```python
from build123d import *

# Parameters (mm, degrees)
SKETCH1_R               = 30.5
BOSS_EXTRUDE1_DEPTH     = 3
CUT_EXTRUDE1_DEPTH      = 95.663789341
CUT_EXTRUDE1_DEPTH_BACK = 95.663789341
SKETCH10_R              = 4
CUT_EXTRUDE2_DEPTH      = 104.861605143
SKETCH11_R              = 21
CUT_EXTRUDE3_DEPTH      = 93.207554018
FILLET1_R               = 5
FILLET2_R               = 5
FILLET3_R               = 5


with BuildPart() as part:
    # Sketch1 → Boss-Extrude1 (new body)
    with BuildSketch(Plane(origin=(0, 0, 0), x_dir=(1, 0, 0), z_dir=(0, 1, 0))):
        Circle(SKETCH1_R)
        with BuildLine():
            Line((22, 21.124630174), (22, 28.495613698))
            ThreePointArc((22, 28.495613698), (0, 36), (-22, 28.495613698))
            Line((-22, 28.495613698), (-22, 21.124630174))
            ThreePointArc((-22, 21.124630174), (0, 30.5), (22, 21.124630174))
        make_face()
    extrude(amount=BOSS_EXTRUDE1_DEPTH)

    # Sketch2 → Loft1 section 0
    with BuildSketch(Plane(origin=(0, 3, 0), x_dir=(1, 0, 0), z_dir=(0, 1, 0))):
        with BuildLine():
            Line((-22, 21.124630174), (-22, 28.495613698))
            Line((-22, 28.495613698), (-19, 28.495613698))
            Line((-19, 28.495613698), (-19, 19.880895352))
            ThreePointArc((-19, 19.880895352), (0, -27.5), (19, 19.880895352))
            Line((19, 19.880895352), (19, 28.495613698))
            Line((19, 28.495613698), (22, 28.495613698))
            Line((22, 28.495613698), (22, 21.124630174))
            ThreePointArc((22, 21.124630174), (0, -30.5), (-22, 21.124630174))
        make_face()
    # Sketch3 → Loft1 section 1
    with BuildSketch(Plane(origin=(0, 78, 0), x_dir=(1, 0, 0), z_dir=(0, 1, 0))):
        with BuildLine():
            Line((-22, 21.124630174), (-22, 44.124630174))
            Line((-22, 44.124630174), (-19, 44.124630174))
            Line((-19, 44.124630174), (-19, 19.880895352))
            ThreePointArc((-19, 19.880895352), (0, -27.5), (19, 19.880895352))
            Line((19, 19.880895352), (19, 44.124630174))
            Line((19, 44.124630174), (22, 44.124630174))
            Line((22, 44.124630174), (22, 21.124630174))
            ThreePointArc((22, 21.124630174), (0, -30.5), (-22, 21.124630174))
        make_face()
    loft()

    # Sketch9 → Cut-Extrude1 (cut, two sides: drawn at the far end of the back side and taken through both)
    with BuildSketch(Plane(origin=(0, 0, 0), x_dir=(0, 0, -1), z_dir=(1, 0, 0)).offset(-CUT_EXTRUDE1_DEPTH_BACK)):
        Polygon((-30.5, 14), (21.124630174, 78), (-30.5, 78), align=None)
    extrude(amount=CUT_EXTRUDE1_DEPTH + CUT_EXTRUDE1_DEPTH_BACK, mode=Mode.SUBTRACT)

    # Sketch10 → Cut-Extrude2 (cut, through all)
    with BuildSketch(Plane.ZY.offset(22)):
        with Locations((-29.124630174, 70)):
            Circle(SKETCH10_R)
    extrude(amount=-CUT_EXTRUDE2_DEPTH, mode=Mode.SUBTRACT)

    # Sketch11 → Cut-Extrude3 (cut, through all)
    with BuildSketch(Plane(origin=(0, 3, 0), x_dir=(1, 0, 0), z_dir=(0, 1, 0))):
        with Locations(Location((0, 0, 0), (0, 0, 270))):
            Circle(SKETCH11_R)
    extrude(amount=-CUT_EXTRUDE3_DEPTH, mode=Mode.SUBTRACT)

    # Fillet1
    fillet1_edges = [part.edges().sort_by_distance(p)[0] for p in [
        (-20.5, 78, -44.124630174),
        (20.5, 78, -44.124630174),
    ]]
    fillet(fillet1_edges, radius=FILLET1_R)

    # Fillet2
    fillet2_edges = [part.edges().sort_by_distance(p)[0] for p in [
        (-20.5, 78, -21.124630174),
        (20.5, 78, -21.124630174),
    ]]
    fillet(fillet2_edges, radius=FILLET2_R)

    # Fillet3
    fillet3_edges = [part.edges().sort_by_distance(p)[0] for p in [
        (19, 39.716879031, -19.880895352),
        (-19, 39.716879031, -19.880895352),
        (22, 38.695702002, -21.124630174),
        (-22, 38.695702002, -21.124630174),
    ]]
    fillet(fillet3_edges, radius=FILLET3_R)


solid = part.part
```
Check sheet for the modelled part. Datum: model origin and axes. Units: mm. A direction names the side the tool comes from. Round coordinates to 2 decimals unless told otherwise and drop trailing zeros. Loops run counter-clockwise (first coordinate to the right, second up) from the corner with the lowest first, then second, coordinate; pieces in that order, holes last. Notation, with made-up numbers: (25, 82.5) -> (30, 82.5) arc R27 ccw to (30, 102.5) -> close; hole circle Ø4 at (-20, -31.75). An arc over 180 degrees is marked (long way). Write item = value, one per line. Start each with the question number.
1) Set-up check for faces 1 (the flat face through (-22, 48, -30)), 2 (the cylindrical face through (23.06, 23.45, 14.98)), 3 (the cylindrical face through (-20.661, 77.524, -21.387)), 4 (the cylindrical face through (0, 1, -36)), 5 (the flat face through (22, 48, -30)): record each of +Z, -Z, +X, -X, +Y, -Y from which the full face is reachable in a straight line by a thin tool's end or side.
2) Sectioned sample at D-D, the plane y = 70. State how many separate pieces and enclosed holes the cut face has, plus the area to 3 significant figures.
3) Gauge pin test, flat ends, axial feed: pin 1 Ø6 at (x, y) = (-15.5, 17) entering from -Z; pin 2 Ø13 at (y, z) = (70, -29.12) entering from +X; pin 3 Ø8 at (y, z) = (57, -10.5) entering from +X. Record the tip position at first contact, or that the pin passes through.
4) Release check for a two-part mould opening along Z. For faces 6 (the flat face through (12, 3, -19)), 7 (the cylindrical face through (6.31, 1.52, 20.03)), 8 (the flat face through (-14, 0, -18)), 9 (the cylindrical face through (20.5, 76.1, -41.9)) record: released by +Z, released by -Z, zero draft, split by the parting line, or undercut.
5) Sectioned sample at A-A, the plane z = 11. Record the cut outline in (x, y), plus the area to 3 significant figures.
6) Sectioned sample at C-C, the plane z = 0. Record the cut outline in (x, y).
7) Sectioned sample at B-B, the plane x = 12. Record the cut outline in (y, z), plus the area to 3 significant figures.
8) Thickness scan on probe 1 along X at (y, z) = (26.5, 0); probe 2 along X at (y, z) = (4, -24.5); probe 3 along Z at (x, y) = (-22.5, 5). Record the ranges inside material, lowest first.
Results are:
q1.face_1 = -Z, -X, +Y, -Y
q1.face_2 = +Y
q1.face_3 = +Z, +X, -X, +Y
q1.face_4 = -Z, -Y
q1.face_5 = -Z, +X, +Y, -Y
q2.separate_pieces = 4
q2.enclosed_holes = 0
q2.area = 128 mm^2
q3.pin_1 = 20.35
q3.pin_2 = 22.02
q3.pin_3 = 29.8
q4.face_6 = undercut
q4.face_7 = undercut
q4.face_8 = zero draft
q4.face_9 = released by -Z
q5.outline = (-28.45, 0) -> (-17.89, 0) -> (-17.89, 3) -> (-25.2, 3) -> (-25.2, 38.17) -> (-28.45, 38.17) -> close; (17.89, 0) -> (28.45, 0) -> (28.45, 38.17) -> (25.2, 38.17) -> (25.2, 3) -> (17.89, 3) -> close
q5.area = 292 mm^2
q6.outline = (-30.5, 0) -> (-21, 0) -> (-21, 3) -> (-27.5, 3) -> (-27.5, 51.81) -> (-30.5, 51.81) -> close; (21, 0) -> (30.5, 0) -> (30.5, 51.81) -> (27.5, 51.81) -> (27.5, 3) -> (21, 3) -> close
q7.outline = (0, -33.94) -> (3, -33.94) -> (3, -17.23) -> (0, -17.23) -> close; (0, 17.23) -> (3, 17.23) -> (3, 24.74) -> (21.14, 24.74) -> (17.05, 28.04) -> (0, 28.04) -> close
q7.area = 136 mm^2
q8.probe_1 = -30.5 to -27.5, 27.5 to 30.5
q8.probe_2 = -22 to -19, 19 to 22
q8.probe_3 = -20.87 to -15.81, 15.81 to 20.59
